Verification items for the finished model (mm, model axes). Face numbers are marked on the shaded views. A direction names the side the tool comes from. Give positions to 0.01 mm unless a question says otherwise; leave off trailing zeros. Order: outer loops, then holes, each group sorted by start corner. A loop starts at its lowest first (then second) coordinate and runs counter-clockwise, first axis right, second up. Notation, with made-up numbers: (79.25, 20) -> (130.25, 20) arc R13 ccw to (130.25, 32) -> close; hole circle Ø2 at (2, -14). An arc over 180 degrees is marked (long way). Return JSON: item names as keys, results as strings. Group by question number.
(1) Tool access check on the marked faces 1, 2 and 3. Record the directions out of +Z, -Z, +X, -X, +Y, -Y that give a thin tool (end or side, any length) a straight path to the whole face; none if there is none.
(2) Cross-section at C-C on x = -51. Enter the section's corners in (y, z), then the cut area to 3 significant figures.
(3) Depth check by flat-ended pin: pin 1 Ø1 at (x, y) = (-21.5, -10) entering from +Z; pin 2 Ø5 at (y, z) = (-8.5, 30.5) entering from -X; pin 3 Ø0.8 at (x, z) = (-62, 33) entering from -Y. Enter the tip coordinate at first touch or a pass-through.
(4) Cross-section at B-B on z = 6. Enter the section's corners in (x, y).
(5) Release check for a two-part mould opening along X. For the marked faces 4, 5 and 6 record: pulls with the +X half, pulls with the -X half, needs draft (parallel to the pull), parting line crosses it, or undercut.
(6) Cross-section at D-D on z = 36.5. Enter the section's corners in (x, y), then the cut area to 3 significant figures.
(7) Cross-section at A-A on x = -28.5. Enter the section's corners in (y, z), then the cut area to 4 significant figures.
(8) Thickness scan on line 1 along X through (y, z) = (-8, 41.5); line 2 along Y through (x, z) = (-59.5, 1); line 3 along Y through (x, z) = (-39, 24.5). Record the ranges inside material, lowest first.
from build123d import *

# Parameters (mm, degrees)
F1_W        = 14
F1_H        = 1.5
F1_R        = 1.5
F2_DEPTH    = 1.5
F3_DEPTH    = 14
F4_DEPTH    = 50
F5_R        = 5
F6_T1_DEPTH = 1.5
F6_T3_DEPTH = 11.9
F6_T5_DEPTH = 1.5


# Not quite as in the source:
# - a fillet or chamfer that OpenCascade refuses, or shapes differently, is made with other operations: its cross-section is extruded or revolved along the edge and cut away or added
# - a feature names something its author has since deleted; it is built from what else it names


with BuildPart() as f2:
    # F1 (on Top) → F2 (new body)
    with BuildSketch(Plane.XY):
        Polygon((-61.5, -10.4), (-61.5, -1.5), (-1.5, -1.5), (-1.5, -10.4), (0, -10.4), (0, 0), (-63, 0), (-63, -10.4), align=None)
        Polygon((-38.5, -10.4), (-61.5, -10.4), (-63, -10.4), (-63, -11.9), (-38.5, -11.9), align=None)
        with Locations((-31.5, -11.15)):
            Rectangle(F1_W, F1_H)
        Polygon((0, -10.4), (-1.5, -10.4), (-24.5, -10.4), (-24.5, -11.9), (0, -11.9), align=None)
        Polygon((-1.5, -1.5), (-61.5, -1.5), (-61.5, -10.4), (-38.5, -10.4), (-24.5, -10.4), (-1.5, -10.4), align=None)
        with BuildLine():
            ThreePointArc((-37.5, -4.45), (-36.9142135624, -3.0357864376), (-35.5, -2.45))
            Line((-35.5, -2.45), (-27.5, -2.45))
            ThreePointArc((-27.5, -2.45), (-26.0857864376, -3.0357864376), (-25.5, -4.45))
            Line((-25.5, -4.45), (-25.5, -7.45))
            ThreePointArc((-25.5, -7.45), (-26.0857864376, -8.8642135624), (-27.5, -9.45))
            Line((-27.5, -9.45), (-35.5, -9.45))
            ThreePointArc((-35.5, -9.45), (-36.9142135624, -8.8642135624), (-37.5, -7.45))
            Line((-37.5, -7.45), (-37.5, -4.45))
        make_face(mode=Mode.SUBTRACT)
        with BuildLine():
            Line((-63, -11.9), (-63, -10.4))
            Line((-63, -10.4), (-63, 0))
            Line((-63, 0), (-66, 0))
            ThreePointArc((-66, 0), (-71.95, -5.95), (-66, -11.9))
            Line((-66, -11.9), (-63, -11.9))
        make_face()
        with Locations((-67.45, -5.95)):
            Circle(F1_R, mode=Mode.SUBTRACT)
        with BuildLine():
            Line((0, 0), (0, -10.4))
            Line((0, -10.4), (0, -11.9))
            Line((0, -11.9), (3, -11.9))
            ThreePointArc((3, -11.9), (8.95, -5.95), (3, 0))
            Line((3, 0), (0, 0))
        make_face()
        with Locations((4.45, -5.95)):
            Circle(F1_R, mode=Mode.SUBTRACT)
    extrude(amount=-F2_DEPTH)

    # F1 (on Top) → F3 (join)
    with BuildSketch(Plane.XY):
        Polygon((0, -10.4), (-1.5, -10.4), (-24.5, -10.4), (-24.5, -11.9), (0, -11.9), align=None)
        Polygon((-38.5, -10.4), (-61.5, -10.4), (-63, -10.4), (-63, -11.9), (-38.5, -11.9), align=None)
    extrude(amount=F3_DEPTH)

    # F1 (on Top) → F4 (join)
    with BuildSketch(Plane.XY):
        Polygon((-61.5, -10.4), (-61.5, -1.5), (-1.5, -1.5), (-1.5, -10.4), (0, -10.4), (0, 0), (-63, 0), (-63, -10.4), align=None)
    extrude(amount=F4_DEPTH)

    # F5
    f5_edges = [f2.edges().sort_by_distance(p)[0] for p in [
        (-62.25, -10.4, 50),
        (-0.75, -10.4, 50),
        (-24.5, -11.15, 14),
        (-38.5, -11.15, 14),
    ]]
    fillet(f5_edges, radius=F5_R)

    # F6: fillet of radius 1.5 on 4 edges, made by hand

    # F6_s2 → F6_t1 (join)
    with BuildSketch(Plane.YZ.offset(-63)):
        with BuildLine():
            ThreePointArc((-10.4, 15.5), (-10.8393398282, 14.4393398282), (-11.9, 14))
            Line((-11.9, 14), (-10.4, 14))
            Line((-10.4, 14), (-10.4, 15.5))
        make_face()
    extrude(amount=F6_T1_DEPTH)

    # F6_s4 → F6_t3 (join)
    with BuildSketch(Plane.XZ):
        with BuildLine():
            ThreePointArc((-63, 1.5), (-63.4393398282, 0.4393398282), (-64.5, 0))
            Line((-64.5, 0), (-63, 0))
            Line((-63, 0), (-63, 1.5))
        make_face()
        with BuildLine():
            ThreePointArc((0, 1.5), (0.4393398282, 0.4393398282), (1.5, 0))
            Line((1.5, 0), (0, 0))
            Line((0, 0), (0, 1.5))
        make_face()
    extrude(amount=F6_T3_DEPTH)

    # F6_s6 → F6_t5 (join)
    with BuildSketch(Plane.YZ.offset(-1.5)):
        with BuildLine():
            ThreePointArc((-10.4, 15.5), (-10.8393398282, 14.4393398282), (-11.9, 14))
            Line((-11.9, 14), (-10.4, 14))
            Line((-10.4, 14), (-10.4, 15.5))
        make_face()
    extrude(amount=F6_T5_DEPTH)


solid = f2.part
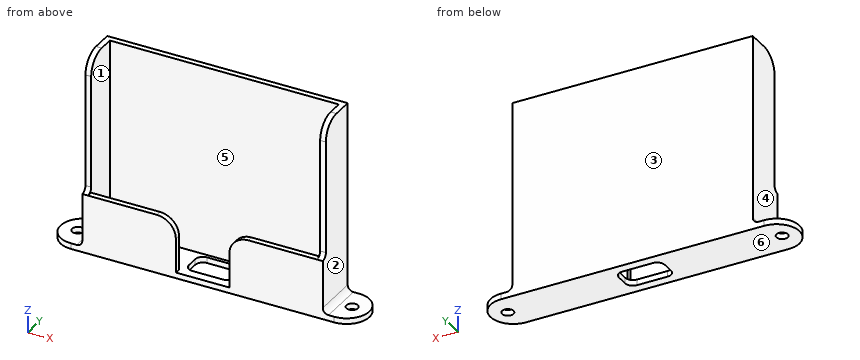
Verdict:
{
 "1": {"face 1": "+Z", "face 2": "+Z, +X, +Y, -Y", "face 3": "+Z, -Z, +X, -X, +Y"},
 "2": {"outline": "(-11.9, -1.5) -> (0, -1.5) -> (0, 50) -> (-1.5, 50) -> (-1.5, 0) -> (-10.4, 0) -> (-10.4, 14) -> (-11.9, 14) -> close", "area": "114 mm²"},
 "3": {"pin 1": "z = 13.7", "pin 2": "x = -63", "pin 3": "y = -10.4"},
 "4": {"outline": "(-63, -11.9) -> (-38.5, -11.9) -> (-38.5, -10.4) -> (-61.5, -10.4) -> (-61.5, -1.5) -> (-1.5, -1.5) -> (-1.5, -10.4) -> (-24.5, -10.4) -> (-24.5, -11.9) -> (0, -11.9) -> (0, 0) -> (-63, 0) -> close"},
 "5": {"face 4": "pulls with the -X half", "face 5": "undercut", "face 6": "needs draft"},
 "6": {"outline": "(-63, -10.4) -> (-61.5, -10.4) -> (-61.5, -1.5) -> (-1.5, -1.5) -> (-1.5, -10.4) -> (0, -10.4) -> (0, 0) -> (-63, 0) -> close", "area": "121 mm²"},
 "7": {"outline": "(-11.9, -1.5) -> (-9.45, -1.5) -> (-9.45, 0) -> (-11.9, 0) -> close; (-2.45, -1.5) -> (0, -1.5) -> (0, 50) -> (-1.5, 50) -> (-1.5, 0) -> (-2.45, 0) -> close", "area": "82.35 mm²"},
 "8": {"line 1": "-63 to -61.5, -1.5 to 0", "line 2": "-11.9 to -10.4, -1.5 to 0", "line 3": "-1.5 to 0"}
}
